Autodesk Inventor part; units mm, degrees
ref_plane "YZ Plane" through (0, 0, 0) normal (1, 0, 0) x (0, 1, 0)
ref_plane "XZ Plane" through (0, 0, 0) normal (0, 1, 0) x (-1, 0, 0)
ref_plane "XY Plane" through (0, 0, 0) normal (0, 0, 1) x (1, 0, 0)
sketch "スケッチ1" plane through (0, 0, 0) normal (0, 0, 1) x (1, 0, 0)
  line L0 (-16, -16) -> (16, -16)
  line L1 (16, -16) -> (16, 16)
  line L2 (16, 16) -> (-16, 16)
  line L3 (-16, 16) -> (-16, -16)
  line L4 (-16, -16) -> (16, 16) construction
  line L5 (16, -16) -> (-16, 16) construction
  line L6 (-14.4, 14.4) -> (14.4, 14.4)
  line L7 (14.4, 14.4) -> (14.4, -14.4)
  line L8 (14.4, -14.4) -> (-14.4, -14.4)
  line L9 (-14.4, -14.4) -> (-14.4, 14.4)
  point P0 (0, 0)
  dimension "d0" = 32
  dimension "d1" = 32
  dimension "d2" = 1.6
extrude "押し出し1" add sketch "スケッチ1" along normal blind 92.5
properties part number "PipeB"
Design review of the part built by this model. Coordinates are the model's own, in mm. A direction names the side the tool comes from. Give positions to 0.01 mm unless a question says otherwise; leave off trailing zeros. Order: outer loops, then holes, each group sorted by start corner. A loop starts at its lowest first (then second) coordinate and runs counter-clockwise, first axis right, second up. Notation, with made-up numbers: (26, -21) - (47, -21) arc R20 ccw to (47, -12) - close; hole circle Ø5 at (63, 43). An arc over 180 degrees is marked (long way). Use CSV: the item, a comma, the result in double quotes. Start each with the question number.
Q1. Take a section at C-C (z = 22.5). State the section outline as (x, y) points.
Q2. Take a section at A-A (x = -1.5). State the section outline as (y, z) points.
Q3. For line 1 (Y direction, x = 13, z = 76), list the stretches that pass through material, from the lowest coordinate up.
Q4. Machinability: for faces 1 (the face through (0, 14.4, 46)), 2 (the face through (0, -16, 46)), which of the approach directions +Z, -Z, +X, -X, +Y, -Y give a long, thin tool a straight path to every point of the face, cutting with its end or side? Answer none if there is none.
Q5. Draft analysis for pull direction Y (two halves, no side actions). For faces 3 (the face through (14.4, 0, 46)), 4 (the face through (16, 0, 46)), 5 (the face through (0, 16, 46)), state which applies: pulls with the +Y half, pulls with the -Y half, needs draft (parallel to the pull), parting line crosses it, or undercut.
Calculated:
1,outline,"(-16, -16) - (16, -16) - (16, 16) - (-16, 16) - close; hole (-14.4, -14.4) - (14.4, -14.4) - (14.4, 14.4) - (-14.4, 14.4) - close"
2,outline,"(-16, 0) - (-14.4, 0) - (-14.4, 92.5) - (-16, 92.5) - close; (14.4, 0) - (16, 0) - (16, 92.5) - (14.4, 92.5) - close"
3,line 1,"y = -16 to -14.4, 14.4 to 16"
4,face 1,"+Z, -Z"
4,face 2,"+Z, -Z, +X, -X, -Y"
5,face 3,"undercut"
5,face 4,"needs draft"
5,face 5,"pulls with the +Y half"
